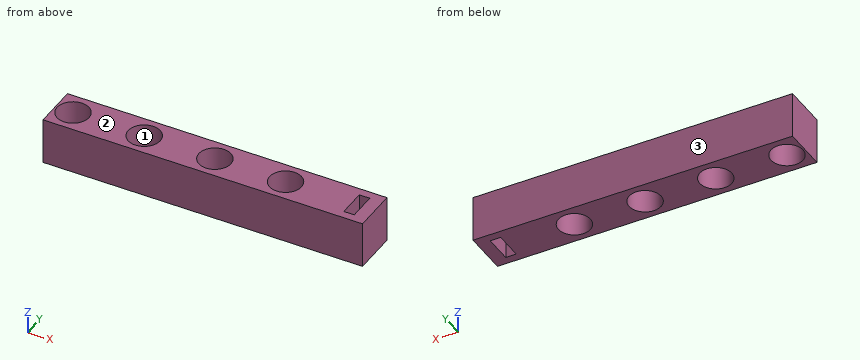
```python
from build123d import *

# Parameters (mm, degrees)
SKIZZE1_W                        = 180
SKIZZE1_H                        = 25
AUFSATZ_LINEAR_AUSTRAGEN1_DEPTH  = 26
F_18_0_18_DURCHMESSER_BOHRUNG2_D = 18
SKIZZE9_W                        = 5.897581214
SKIZZE9_H                        = 15.867301838
SCHNITT_LINEAR_AUSTRAGEN1_DEPTH  = 27


with BuildPart() as part:
    # Skizze1 → Aufsatz-Linear austragen1 (new body)
    with BuildSketch(Plane.XY):
        with Locations((90, 12.5)):
            Rectangle(SKIZZE1_W, SKIZZE1_H)
    extrude(amount=AUFSATZ_LINEAR_AUSTRAGEN1_DEPTH)

    # Ø18.0 (18) Durchmesser Bohrung2 (through all)
    with Locations(Plane.XY.offset(26)):
        with Locations((9.995618269, 12.5), (50.121303026, 12.5), (89.934725645, 12.5), (129.748148264, 12.5)):
            Hole(F_18_0_18_DURCHMESSER_BOHRUNG2_D / 2)

    # Skizze9 → Schnitt-Linear austragen1 (cut, through all)
    with BuildSketch(Plane.XY.offset(26)):
        with Locations((169.861933283, 12.524643843)):
            Rectangle(SKIZZE9_W, SKIZZE9_H)
    extrude(amount=-SCHNITT_LINEAR_AUSTRAGEN1_DEPTH, mode=Mode.SUBTRACT)


solid = part.part
```
Input: part model. Units: mm. Frame: model coordinates. Face numbers are marked on the shaded views. Coordinates: 2 decimals unless noted, no trailing zeros. Loops run counter-clockwise (first coordinate to the right, second up) from the corner with the lowest first, then second, coordinate; pieces in that order, holes last. Notation, with made-up numbers: (-22, 37.5) - (37, 37.5) arc R21 cw to (37, 61.5) - close; hole circle Ø4 at (-15, 49). An arc over 180 degrees is marked (long way). Answer in a Markdown table with one row per item.
(1) Cut plane A-A on z = 11.25. Output: boundary loops of the cut face in (x, y).
Model answer:
| item | result |
|---|---|
| outline | (0, 0) - (180, 0) - (180, 25) - (0, 25) - close; hole circle Ø18 at (10, 12.5); hole circle Ø18 at (50.12, 12.5); hole circle Ø18 at (89.93, 12.5); hole circle Ø18 at (129.75, 12.5); hole (166.91, 4.59) - (172.81, 4.59) - (172.81, 20.46) - (166.91, 20.46) - close |
(2) Cut plane B-B on y = 12.5. Output: boundary loops of the cut face in (x, z).
Model answer:
| item | result |
|---|---|
| outline | (0, 0) - (1, 0) - (1, 26) - (0, 26) - close; (19, 0) - (41.12, 0) - (41.12, 26) - (19, 26) - close; (59.12, 0) - (80.93, 0) - (80.93, 26) - (59.12, 26) - close; (98.93, 0) - (120.75, 0) - (120.75, 26) - (98.93, 26) - close; (138.75, 0) - (166.91, 0) - (166.91, 26) - (138.75, 26) - close; (172.81, 0) - (180, 0) - (180, 26) - (172.81, 26) - close |
(3) Cut plane D-D on x = 86. Output: boundary loops of the cut face in (y, z).
Model answer:
| item | result |
|---|---|
| outline | (0, 0) - (4.41, 0) - (4.41, 26) - (0, 26) - close; (20.59, 0) - (25, 0) - (25, 26) - (20.59, 26) - close |
(4) Material intervals for L1, parallel to X at y = 13.25, z = 13.5; L2, parallel to X at y = 19, z = 10.75; L3, parallel to Y at x = 57, z = 21.5, sorted ascending. Write a range as from..to.
Model answer:
| item | result |
|---|---|
| L1 | x = 0..1.03, 18.96..41.15, 59.09..80.97, 98.9..120.78, 138.72..166.91, 172.81..180 |
| L2 | x = 0..3.77, 16.22..43.9, 56.35..83.71, 96.16..123.52, 135.97..166.91, 172.81..180 |
| L3 | y = 0..6.7, 18.3..25 |
(5) Mould query, pull axis Y, two halves, no side actions, for the marked faces 1, 2 and 3. Classes: pulls with the +Y half, pulls with the -Y half, needs draft (parallel to the pull), parting line crosses it, or undercut.
Model answer:
| item | result |
|---|---|
| face 1 | undercut |
| face 2 | needs draft |
| face 3 | pulls with the +Y half |
(6) Cut plane C-C on x = 136. Output: boundary loops of the cut face in (y, z), plus the area to 3 significant figures.
Model answer:
| item | result |
|---|---|
| outline | (0, 0) - (6.03, 0) - (6.03, 26) - (0, 26) - close; (18.97, 0) - (25, 0) - (25, 26) - (18.97, 26) - close |
| area | 313 mm² |
(7) Pin query (flat end, axial travel): P1, Ø6, axis at x = 58, y = 8, coming from the -Z side; P2, Ø11, axis at x = 10, y = 12.5, coming from the -Z side. Return the tip coordinate at first contact, or that it passes through.
Model answer:
| item | result |
|---|---|
| P1 | stops at z = 0 |
| P2 | passes through |
